```python
from build123d import *

# Parameters (mm, degrees)
SKETCH_1_W                      = 15
SKETCH_1_H                      = 15
EXTRUDE_1_DEPTH                 = 5
SKETCH_2_W                      = 3
SKETCH_2_H                      = 3
EXTRUDE_2_DEPTH                 = 1
EXTRUDE_3_DEPTH                 = 2
EXTRUDE_3_DEPTH_BACK            = 2
CUT_EXTRUDE_1_REACH             = 13.726
CUT_EXTRUDE_1_DIRECTION_2_REACH = 13.726
CUT_EXTRUDE_2_REACH             = 19.5
FILLET_1_R                      = 0.1
FILLET_2_R                      = 0.2


with BuildPart() as part:
    # 草图1 → 凸台-拉伸1 (new body)
    with BuildSketch(Plane.XY):
        Rectangle(SKETCH_1_W, SKETCH_1_H)
    extrude(amount=-EXTRUDE_1_DEPTH)

    # 草图2 → 凸台-拉伸2 (add)
    with BuildSketch(Plane.XY):
        Rectangle(SKETCH_2_W, SKETCH_2_H)
    extrude(amount=EXTRUDE_2_DEPTH)

    # 草图3 → 凸台-拉伸3 (add, two sides: drawn at the far end of the back side and taken through both)
    with BuildSketch(Plane(origin=(0, 0, 0), x_dir=(1, 0, 0), z_dir=(0, 1, 0)).offset(-EXTRUDE_3_DEPTH_BACK)):
        with BuildLine():
            Line((-1.95, -2.5), (1.95, -2.5))
            Line((1.95, -2.5), (1.95, -1.555590279))
            ThreePointArc((1.95, -1.555590279), (1.780042303, -1.088161527), (1.5, -0.677124344))
            Line((1.5, -0.677124344), (-1.5, -0.677124344))
            ThreePointArc((-1.5, -0.677124344), (-1.780042303, -1.088161527), (-1.95, -1.555590279))
            Line((-1.95, -1.555590279), (-1.95, -2.5))
        make_face()
    extrude(amount=EXTRUDE_3_DEPTH + EXTRUDE_3_DEPTH_BACK)

    # 草图4 → 切除-拉伸1 (cut, up to next)
    with BuildSketch(Plane(origin=(0, 0, 0), x_dir=(0, 0, -1), z_dir=(1, 0, 0)), mode=Mode.PRIVATE) as cut_extrude_1_sk1:
        with BuildLine():
            Line((-2.5, 1.95), (-1.555590279, 1.95))
            ThreePointArc((-1.555590279, 1.95), (-1.088161527, 1.780042303), (-0.677124344, 1.5))
            Line((-0.677124344, 1.5), (-0.677124344, 2))
            Line((-0.677124344, 2), (-2.5, 2))
            Line((-2.5, 2), (-2.5, 1.95))
        make_face()
    cut_extrude_1_tool1 = extrude(cut_extrude_1_sk1.sketch, amount=-CUT_EXTRUDE_1_REACH, mode=Mode.PRIVATE) & part.part
    # 草图4 → 切除-拉伸1 (cut, up to next)
    with BuildSketch(Plane(origin=(0, 0, 0), x_dir=(0, 0, -1), z_dir=(1, 0, 0)), mode=Mode.PRIVATE) as cut_extrude_1_sk2:
        with BuildLine():
            Line((-2.5, -2), (-0.677124344, -2))
            Line((-0.677124344, -2), (-0.677124344, -1.5))
            ThreePointArc((-0.677124344, -1.5), (-1.088161527, -1.780042303), (-1.555590279, -1.95))
            Line((-1.555590279, -1.95), (-2.5, -1.95))
            Line((-2.5, -1.95), (-2.5, -2))
        make_face()
    cut_extrude_1_tool2 = extrude(cut_extrude_1_sk2.sketch, amount=-CUT_EXTRUDE_1_REACH, mode=Mode.PRIVATE) & part.part
    add(cut_extrude_1_tool1.solids().sort_by_distance((0, 1.873038, 1.175075))[0], mode=Mode.SUBTRACT)
    add(cut_extrude_1_tool2.solids().sort_by_distance((0, -1.873038, 1.175075))[0], mode=Mode.SUBTRACT)

    # 草图4 → 切除-拉伸1 direction 2 (cut, up to next)
    with BuildSketch(Plane(origin=(0, 0, 0), x_dir=(0, 0, -1), z_dir=(1, 0, 0)), mode=Mode.PRIVATE) as cut_extrude_1_direction_2_sk1:
        with BuildLine():
            Line((-2.5, 1.95), (-1.555590279, 1.95))
            ThreePointArc((-1.555590279, 1.95), (-1.088161527, 1.780042303), (-0.677124344, 1.5))
            Line((-0.677124344, 1.5), (-0.677124344, 2))
            Line((-0.677124344, 2), (-2.5, 2))
            Line((-2.5, 2), (-2.5, 1.95))
        make_face()
    cut_extrude_1_direction_2_tool1 = extrude(cut_extrude_1_direction_2_sk1.sketch, amount=CUT_EXTRUDE_1_DIRECTION_2_REACH, mode=Mode.PRIVATE) & part.part
    # 草图4 → 切除-拉伸1 direction 2 (cut, up to next)
    with BuildSketch(Plane(origin=(0, 0, 0), x_dir=(0, 0, -1), z_dir=(1, 0, 0)), mode=Mode.PRIVATE) as cut_extrude_1_direction_2_sk2:
        with BuildLine():
            Line((-2.5, -2), (-0.677124344, -2))
            Line((-0.677124344, -2), (-0.677124344, -1.5))
            ThreePointArc((-0.677124344, -1.5), (-1.088161527, -1.780042303), (-1.555590279, -1.95))
            Line((-1.555590279, -1.95), (-2.5, -1.95))
            Line((-2.5, -1.95), (-2.5, -2))
        make_face()
    cut_extrude_1_direction_2_tool2 = extrude(cut_extrude_1_direction_2_sk2.sketch, amount=CUT_EXTRUDE_1_DIRECTION_2_REACH, mode=Mode.PRIVATE) & part.part
    add(cut_extrude_1_direction_2_tool1.solids().sort_by_distance((0, 1.873038, 1.175075))[0], mode=Mode.SUBTRACT)
    add(cut_extrude_1_direction_2_tool2.solids().sort_by_distance((0, -1.873038, 1.175075))[0], mode=Mode.SUBTRACT)

    # 草图5 → 切除-拉伸2 (cut, up to next)
    with BuildSketch(Plane.XZ.offset(7.5), mode=Mode.PRIVATE) as cut_extrude_2_sk1:
        with BuildLine():
            Line((-1.5, -5), (-1.5, -4.322875656))
            ThreePointArc((-1.5, -4.322875656), (-1.870828693, -3.707106781), (-2, -3))
            Line((-2, -3), (-2, -2.2))
            Line((-2, -2.2), (2, -2.2))
            Line((2, -2.2), (2, -3))
            ThreePointArc((2, -3), (1.870828693, -3.707106781), (1.5, -4.322875656))
            Line((1.5, -4.322875656), (1.5, -5))
            Line((1.5, -5), (-1.5, -5))
        make_face()
    cut_extrude_2_tool1 = extrude(cut_extrude_2_sk1.sketch, amount=-CUT_EXTRUDE_2_REACH, mode=Mode.PRIVATE) & part.part
    add(cut_extrude_2_tool1.solids().sort_by_distance((0, -7.5, -3.51237))[0], mode=Mode.SUBTRACT)

    # 圆角1
    fillet_1_edges = [part.edges().sort_by_distance(p)[0] for p in [
        (-1.95, 0, 2.5),
        (1.95, 0, 2.5),
        (0, -1.95, 2.5),
        (0, 1.95, 2.5),
    ]]
    fillet(fillet_1_edges, radius=FILLET_1_R)

    # 圆角2
    fillet_2_edges = [part.edges().sort_by_distance(p)[0] for p in [
        (7.5, 0, -5),
        (4.5, 7.5, -5),
        (-7.5, 0, -5),
        (0, 7.5, 0),
        (7.5, 0, 0),
        (0, -7.5, 0),
        (-7.5, 0, 0),
        (-4.5, -7.5, -5),
        (-7.5, 7.5, -2.5),
        (7.5, 7.5, -2.5),
        (7.5, -7.5, -2.5),
        (-7.5, -7.5, -2.5),
        (-4.5, 7.5, -5),
        (4.5, -7.5, -5),
        (1.5, 0, -5),
        (-1.5, 0, -5),
    ]]
    fillet(fillet_2_edges, radius=FILLET_2_R)


solid = part.part
```
Model file for the job. Use its own axes, mm. A direction names the side the tool comes from. Give positions to 0.01 mm unless a question says otherwise; leave off trailing zeros. Order: outer loops, then holes, each group sorted by start corner. A loop starts at its lowest first (then second) coordinate and runs counter-clockwise, first axis right, second up.
1) Pin check, flat tips, straight feed: pin 1 (0.9 mm diameter, centred on y = -0.5, z = 2, fed in from -X); pin 2 (0.5 mm diameter, centred on x = -0.5, z = 0.5, fed in from +Y). Stop position of each tip, or through.
2) Saw through at B-B, the plane y = -3.75. Write the cut outline in (x, z), then the cut area to 3 significant figures.
3) Mould opens along Z. For faces 6 (the flat face through (0, 0, 2.5)), 7 (the cylindrical face through (-1.777, -0.027, 1.082)), 8 (the flat face through (7.5, 0, -2)) say: +Z half, -Z half, draft (parallel to the pull), parting line (faces both ways), or undercut.
4) Saw through at A-A, the plane x = 1.25. Write the cut outline in (y, z), then the cut area to 3 significant figures.
5) 3-axis set-ups, long thin cutter, end or side, ignore diameter. For faces 1 (the cylindrical face through (1.78, -0.03, 1.09)), 2 (the flat face through (0, -1.95, 2)), 3 (the cylindrical face through (1.874, -0.105, -3.698)), 4 (the cylindrical face through (-0.03, 1.78, 1.09)), 5 (the flat face through (-1.95, 0, 2)): which of +Z, -Z, +X, -X, +Y, -Y reach the whole face in a straight line?
6) Wall check: probe 1 along X at (y, z) = (-0.75, -2.5); probe 2 along Z at (x, y) = (6, -4.25); probe 3 along X at (y, z) = (-0.75, -4.5). Give the ranges that are in metal, low to high.
7) Saw through at D-D, the plane x = 5.25. Write the cut outline in (y, z).
8) Saw through at C-C, the plane y = 1.25. Write the cut outline in (x, z).
Computed:
1. pin 1: stops at x = -1.95
1. pin 2: stops at y = 1.56
2. outline: (-7.5, -4.8) arc R0.2 ccw to (-7.3, -5) - (-1.7, -5) arc R0.2 ccw to (-1.5, -4.8) - (-1.5, -4.32) arc R2 cw to (-2, -3) - (-2, -2.2) - (2, -2.2) - (2, -3) arc R2 cw to (1.5, -4.32) - (1.5, -4.8) arc R0.2 ccw to (1.7, -5) - (7.3, -5) arc R0.2 ccw to (7.5, -4.8) - (7.5, -0.2) arc R0.2 ccw to (7.3, 0) - (-7.3, 0) arc R0.2 ccw to (-7.5, -0.2) - close
2. area: 64.8 mm2
3. face 6: +Z half
3. face 7: undercut
3. face 8: draft
4. outline: (-7.5, -2.2) - (7.5, -2.2) - (7.5, -0.2) arc R0.2 ccw to (7.3, 0) - (1.5, 0) - (1.5, 0.68) arc R2 ccw to (1.95, 1.56) - (1.95, 2.4) arc R0.1 ccw to (1.85, 2.5) - (-1.85, 2.5) arc R0.1 ccw to (-1.95, 2.4) - (-1.95, 1.56) arc R2 ccw to (-1.5, 0.68) - (-1.5, 0) - (-7.3, 0) arc R0.2 ccw to (-7.5, -0.2) - close
4. area: 41.8 mm2
5. face 1: +X, +Y, -Y
5. face 2: +Z, +X, -X, -Y
5. face 3: +Y, -Y
5. face 4: +X, -X, +Y
5. face 5: +Z, -X, +Y, -Y
6. probe 1: x = -7.5 to -2, 2 to 7.5
6. probe 2: z = -5 to 0
6. probe 3: x = -7.5 to -1.5, 1.5 to 7.5
7. outline: (-7.5, -4.8) arc R0.2 ccw to (-7.3, -5) - (7.3, -5) arc R0.2 ccw to (7.5, -4.8) - (7.5, -0.2) arc R0.2 ccw to (7.3, 0) - (-7.3, 0) arc R0.2 ccw to (-7.5, -0.2) - close
8. outline: (-7.5, -4.8) arc R0.2 ccw to (-7.3, -5) - (-1.7, -5) arc R0.2 ccw to (-1.5, -4.8) - (-1.5, -4.32) arc R2 cw to (-2, -3) - (-2, -2.2) - (2, -2.2) - (2, -3) arc R2 cw to (1.5, -4.32) - (1.5, -4.8) arc R0.2 ccw to (1.7, -5) - (7.3, -5) arc R0.2 ccw to (7.5, -4.8) - (7.5, -0.2) arc R0.2 ccw to (7.3, 0) - (1.5, 0) - (1.5, 0.68) arc R2 ccw to (1.95, 1.56) - (1.95, 2.4) arc R0.1 ccw to (1.85, 2.5) - (-1.85, 2.5) arc R0.1 ccw to (-1.95, 2.4) - (-1.95, 1.56) arc R2 ccw to (-1.5, 0.68) - (-1.5, 0) - (-7.3, 0) arc R0.2 ccw to (-7.5, -0.2) - close
